```python
from build123d import *

# Parameters (mm, degrees)
SKETCH_1_R      = 1
SKETCH_1_R_2    = 1.5
SKETCH_1_W      = 2.85
SKETCH_1_H      = 5
EXTRUDE_1_DEPTH = 1.4


with BuildPart() as part:
    # Эскиз1 → Бобышка-Вытянуть1 (new, symmetric)
    with BuildSketch(Plane.XY):
        with BuildLine():
            ThreePointArc((175.091334091, 16.644787515), (168.620686799, 13.96455765), (165.940456932, 7.493910359))
            ThreePointArc((165.940456932, 7.493910359), (168.620686797, 1.023263065), (175.091334091, -1.656966802))
            add(Edge.make_bspline(
                [(175.091334091, -1.656966802), (177.330680613, -1.588466601), (181.854695323, -1.455127256), (188.663234462, -1.270383377), (194.423908611, -1.128102082), (197.899847219, -1.04871935), (199.091334091, -1.02226769)],
                knots=[0.704401069, 0.704401069, 0.704401069, 0.704401069, 0.730918775, 0.757971338, 0.785017763, 0.79912389, 0.79912389, 0.79912389, 0.79912389], degree=3))
            Line((199.091334091, -1.02226769), (204.343876183, -6.698358978))
            ThreePointArc((204.343876183, -6.698358978), (205.086913668, -7.019125459), (205.824005665, -6.684923086))
            Line((205.824005665, -6.684923086), (211.091334091, -0.78138581))
            add(Edge.make_bspline(
                [(211.091334091, -0.78138581), (215.029550732, -0.71061193), (221.226120504, -0.611852577), (229.617630172, -0.50292618), (236.087353854, -0.431514192), (241.980776913, -0.376520461), (246.558970011, -0.339535886), (249.120490965, -0.321271242), (250, -0.315)],
                knots=[0.846478182, 0.846478182, 0.846478182, 0.846478182, 0.893099152, 0.919831065, 0.945809917, 0.969680601, 0.989589706, 1, 1, 1, 1], degree=3))
            ThreePointArc((250, -0.315), (250.130477272, 0), (250, 0.315))
            add(Edge.make_bspline(
                [(250, 0.315), (249.15566774, 0.545019818), (246.720175698, 1.208516243), (242.391332083, 2.358339053), (236.849761204, 3.787625364), (230.779918279, 5.298008837), (224.455917947, 6.812866028), (218.030543496, 8.291610632), (211.562405045, 9.719735057), (205.072411509, 11.092374932), (198.567970913, 12.407850726), (192.052369914, 13.665297924), (185.527619973, 14.864093303), (179.872800983, 15.850364437), (176.392239334, 16.431323122), (175.091334091, 16.644787515)],
                knots=[0, 0, 0, 0, 0.0101622, 0.029313053, 0.052011605, 0.076619468, 0.101948061, 0.127526132, 0.153184131, 0.178867888, 0.204557903, 0.230245712, 0.255925967, 0.281594302, 0.296903142, 0.296903142, 0.296903142, 0.296903142], degree=3))
        make_face()
        with Locations((205.091334091, -3.806089643)):
            Circle(SKETCH_1_R, mode=Mode.SUBTRACT)
        with Locations((175.091334091, 7.493910357)):
            Circle(SKETCH_1_R_2, mode=Mode.SUBTRACT)
        with Locations((205.091334091, 4.493910357)):
            Rectangle(SKETCH_1_W, SKETCH_1_H, mode=Mode.SUBTRACT)
    extrude(amount=EXTRUDE_1_DEPTH, both=True)


solid = part.part
```
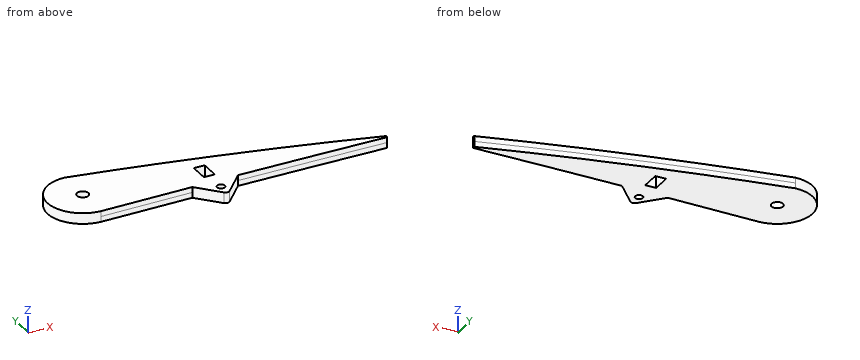
Here's how the part is built. I have some questions about the finished solid (model axes, mm). Give positions to 0.01 mm unless a question says otherwise; leave off trailing zeros. Return JSON: item names as keys, results as strings.
Item 1: Please list where these lines run through material, in increasing order: line 1 (Y direction, x = 174.5, z = -1.15); line 2 (Y direction, x = 182, z = 1.05); line 3 (Y direction, x = 185, z = -0.8).
A:
{"line 1": "y = -1.64 to 6.12, 8.87 to 16.63", "line 2": "y = -1.45 to 15.48", "line 3": "y = -1.37 to 14.95"}
Item 2: Imagine slicing it at A-A on z = -0.8. State how many separate pieces and enclosed holes the cut face has, then the cut area to 3 significant figures.
A:
{"separate pieces": "1", "enclosed holes": "3", "area": "895 mm^2"}
Item 3: I'm going to push flat-ended pins straight in: pin 1 Ø1 at (x, z) = (216.5, 1) entering from +Y; pin 2 Ø1.4 at (y, z) = (3.5, -0.5) entering from -X; pin 3 Ø1 at (x, z) = (213, 0) entering from -Y. Where does each tip first touch, or does it pass through?
A:
{"pin 1": "stops at y = 8.74", "pin 2": "stops at x = 166.55", "pin 3": "stops at y = -0.76"}
